Here's how the part is built. I have some questions about the finished solid (model axes, mm). A direction names the side the tool comes from. Round coordinates to 2 decimals unless told otherwise and drop trailing zeros. Order: outer loops, then holes, each group sorted by start corner. A loop starts at its lowest first (then second) coordinate and runs counter-clockwise, first axis right, second up.
```python
from build123d import *

# Parameters (mm, degrees)
SKETCH_1_R      = 2
EXTRUDE_1_DEPTH = 40
SKETCH_2_R      = 3.25
EXTRUDE_2_DEPTH = 2.2
FILLET_1_R      = 1.5


with BuildPart() as part:
    # 草图1 → 凸台-拉伸1 (new body)
    with BuildSketch(Plane.XY):
        Circle(SKETCH_1_R)
    extrude(amount=EXTRUDE_1_DEPTH)

    # 草图2 → 凸台-拉伸2 (add)
    with BuildSketch(Plane.XY.offset(40)):
        Circle(SKETCH_2_R)
    extrude(amount=EXTRUDE_2_DEPTH)

    # 圆角1
    fillet_1_edges = [part.edges().sort_by_distance(p)[0] for p in [
        (-3.25, 0, 42.2),
    ]]
    fillet(fillet_1_edges, radius=FILLET_1_R)


solid = part.part
```
1. I need wall thicknesses on probe 1 along Y at (x, z) = (0, 15); probe 2 along Y at (x, z) = (0.75, 12); probe 3 along Z at (x, y) = (-1, 2.75). Which ranges of each line are inside material? Lowest first, please.
Evaluation:
probe 1: y = -2 to 2
probe 2: y = -1.85 to 1.85
probe 3: z = 40 to 41.63
2. If we section it at A-A, the plane y = 0: Write out the boundary of the cut face in (x, z).
Evaluation:
outline: (-3.25, 40) - (-2, 40) - (-2, 0) - (2, 0) - (2, 40) - (3.25, 40) - (3.25, 40.7) arc R1.5 ccw to (1.75, 42.2) - (-1.75, 42.2) arc R1.5 ccw to (-3.25, 40.7) - close
3. On a 3-axis mill with a long thin cutter (end or side, diameter ignored), from which of +Z, -Z, +X, -X, +Y, -Y can I reach the whole of each face in a straight line? I mean faces 1 (the flat face through (0, 0, 42.2)), 2 (the flat face through (1, -2, 40)). Say none if no direction works.
Evaluation:
face 1: +Z, +X, -X, +Y, -Y
face 2: -Z
4. I'm going to push flat-ended pins straight in: P1, Ø2, axis at x = -1, z = 7.5, coming from the +Y side; P2, Ø2, axis at x = -0.5, y = -0.5, coming from the -Z side. Where does each tip first touch, or does it pass through?
Evaluation:
P1: stops at y = 2
P2: stops at z = 0
5. If we section it at C-C, the plane z = 14: Write out the boundary of the cut face in (x, y).
Evaluation:
outline: circle Ø4 at (0, 0)
